CAD build for the part. Positions are in the model's coordinates, mm. Give positions to 0.01 mm unless a question says otherwise; leave off trailing zeros. Order: outer loops, then holes, each group sorted by start corner. A loop starts at its lowest first (then second) coordinate and runs counter-clockwise, first axis right, second up. Notation, with made-up numbers: (52, 63.25) -> (76, 63.25) arc R18 ccw to (76, 78.25) -> close; hole circle Ø6 at (19.5, 38.5). An arc over 180 degrees is marked (long way). Use one line per item in the form item = value. Start each with the question number.
1) Drop flat-ended pins along their axis: P1, Ø1, axis at x = 15.5, y = -10.5, coming from the -Z side; P2, Ø3.5, axis at y = -8, z = 19, coming from the +X side. Give the stop position or say it passes through.
2) Cut at B-B, the plane y = -9.5. State how many separate pieces and enclosed holes the cut face has, and give its area (3 significant figures).
3) Cut at A-A, the plane x = 6. Give the cut face in (y, z).
4) Probe line 1 (Z direction, x = -86.5, y = -7.5); line 2 (Z direction, x = 24, y = -0.25); line 3 (Z direction, x = -91, y = -2.75). List the from-to ranges inside material, lowest first.
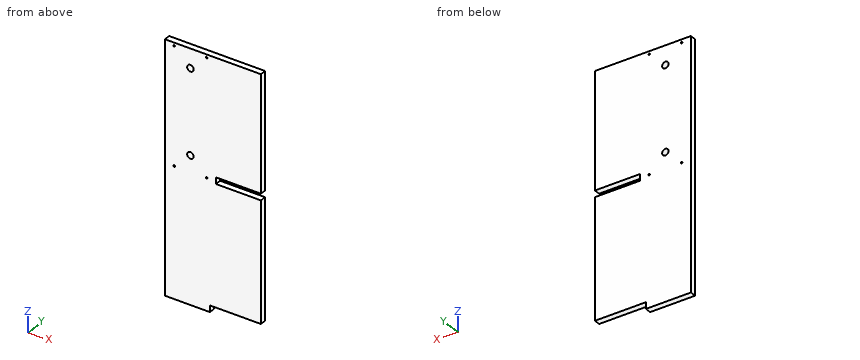
from build123d import *

# Parameters (mm, degrees)
F1_DEPTH = 11.938
F2_R     = 6.35
F2_R_2   = 1.5875
F3_DEPTH = 11.939


with BuildPart() as f1:
    # F0 (on Front) → F1 (new body)
    with BuildSketch(Plane.XZ):
        Polygon((-36.348071, 252.832707), (-136.424071, 252.832707), (-136.424071, -233.005793), (-48.286071, -233.005793), (-48.286071, -220.305793), (51.789929, -220.305793), (51.789929, 13.818707), (-36.348071, 13.818707), (-36.348071, 26.518707), (51.789929, 26.518707), (51.789929, 252.832707), align=None)
    extrude(amount=F1_DEPTH)

    # F2 (on face) → F3 (cut, through all)
    with BuildSketch(Plane.XZ.offset(11.938)):
        with Locations((-86.386071, 215.494707)):
            Circle(F2_R)
        with Locations((-86.386071, 50.394707)):
            Circle(F2_R)
        with Locations((-118.136071, 246.863707)):
            Circle(F2_R_2)
        with Locations((-54.636071, 246.863707)):
            Circle(F2_R_2)
        with Locations((-118.136071, 19.025707)):
            Circle(F2_R_2)
        with Locations((-54.636071, 19.025707)):
            Circle(F2_R_2)
    extrude(amount=-F3_DEPTH, mode=Mode.SUBTRACT)


solid = f1.part
Result:
q1.P1 = -220.31
q1.P2 = -36.35
q2.separate_pieces = 1
q2.enclosed_holes = 6
q2.area = 88,800 mm²
q3.outline = (-11.94, -220.31) -> (0, -220.31) -> (0, 13.82) -> (-11.94, 13.82) -> close; (-11.94, 26.52) -> (0, 26.52) -> (0, 252.83) -> (-11.94, 252.83) -> close
q4.line_1 = -233.01 to 44.05, 56.74 to 209.15, 221.84 to 252.83
q4.line_2 = -220.31 to 13.82, 26.52 to 252.83
q4.line_3 = -233.01 to 46.03, 54.76 to 211.13, 219.86 to 252.83
